```python
from build123d import *

# Parameters (mm, degrees)
F0_W     = 20
F0_H     = 20
F1_DEPTH = 10
F2_R     = 10
F3_DEPTH = 10
F4_R     = 6.828336
F5_DEPTH = 10
F6_SIZE  = 6.8


with BuildPart() as f1:
    # F0 (on Top) → F1 (new body)
    with BuildSketch(Plane.XY):
        Rectangle(F0_W, F0_H)
    extrude(amount=F1_DEPTH)

    # F2 (on face) → F3 (join)
    with BuildSketch(Plane.XY.offset(10)):
        Circle(F2_R)
    extrude(amount=F3_DEPTH)

    # F4 (on face) → F5 (join)
    with BuildSketch(Plane.XY.offset(20)):
        Circle(F4_R)
    extrude(amount=F5_DEPTH)

    # F6
    f6_edges = [f1.edges().sort_by_distance(p)[0] for p in [
        (-6.828336, 0, 30),
    ]]
    chamfer(f6_edges, length=F6_SIZE)


solid = f1.part
```
For this review, take the finished solid that the model builds, in its own axes (mm). A direction names the side the tool comes from. Round coordinates to 2 decimals unless told otherwise and drop trailing zeros. Write each loop counter-clockwise with the first axis right and the second up, starting at its lowest first coordinate (ties: lowest second). Pieces come first, ordered by that corner, then holes. Notation, with made-up numbers: (80.5, 29) - (133.5, 29) arc R8 ccw to (133.5, 44) - close; hole circle Ø1 at (45, 70.5). An arc over 180 degrees is marked (long way). Use CSV: the item, a comma, the result in double quotes.
1) Add section B-B on z = 22.25. Write out the cut boundary in (x, y).
Conclusion:
outline,"circle Ø13.66 at (0, 0)"
2) Wall thickness on line 1 along Z through (x, y) = (4.5, 9); line 2 along Z through (x, y) = (9, -3.25); line 3 along Y through (x, z) = (3.5, 14.75): over which ranges is each line inside the solid? List them lowest first. Write a range as from..to.
Conclusion:
line 1,"z = 0..10"
line 2,"z = 0..20"
line 3,"y = -9.37..9.37"
3) For faces 1 (the flat face through (8, -8, 10)), 2 (the flat face through (8, 8, 10)), 3 (the flat face through (7, -2, 20)), list the 3-axis set-ups (+Z, -Z, +X, -X, +Y, -Y) from which the entire face can be reached by the end or side of a thin tool; tool diameter is ignored.
Conclusion:
face 1,"+Z, +X, -Y"
face 2,"+Z, +X, +Y"
face 3,"+Z"
4) Clearance check with flat-ended pins moving along their axes: pin 1 Ø10 at (x, y) = (4.5, -4.5) entering from +Z; pin 2 Ø1 at (x, y) = (-0.5, -4) entering from +Z; pin 3 Ø6 at (y, z) = (4.5, 13.5) entering from -X. State where each tip first meets the part, or that it passes through.
Conclusion:
pin 1,"stops at z = 28.66"
pin 2,"stops at z = 26.5"
pin 3,"stops at x = -9.89"
5) Add section A-A on x = 8.5. Write out the cut boundary in (y, z), and give its area (3 significant figures).
Conclusion:
outline,"(-10, 0) - (10, 0) - (10, 10) - (5.27, 10) - (5.27, 20) - (-5.27, 20) - (-5.27, 10) - (-10, 10) - close"
area,"305 mm^2"
